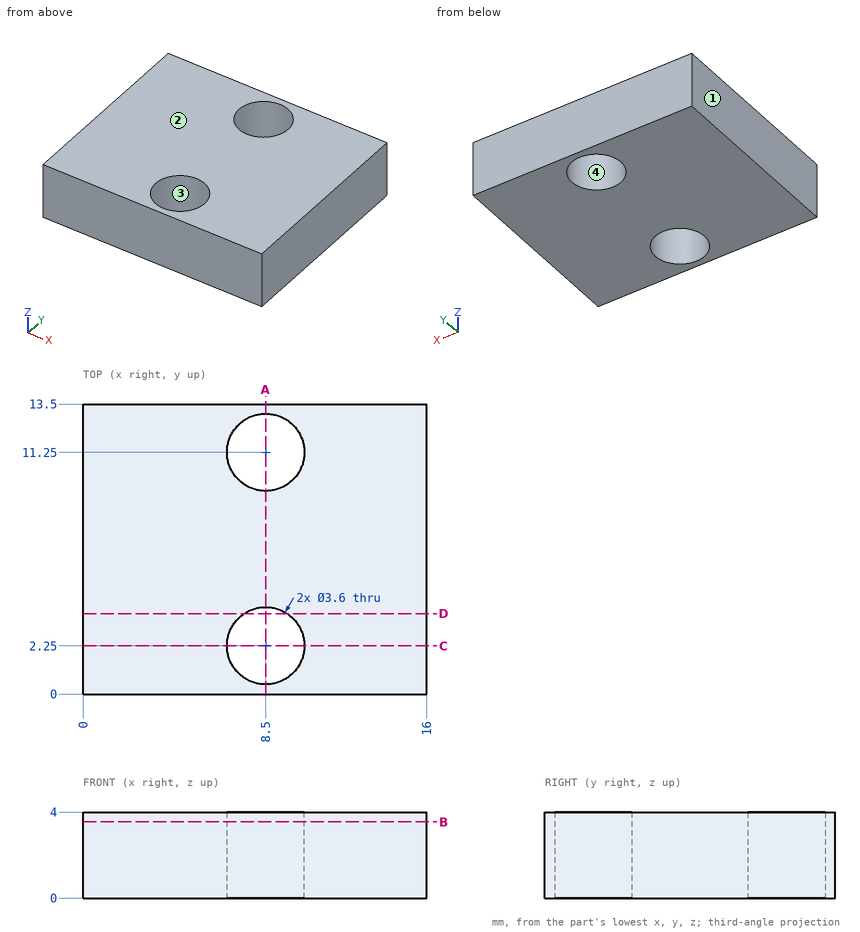
Geometry: see drawing. Coordinates: mm, zero at the bounding-box minimum. Round coordinates to 2 decimals unless told otherwise and drop trailing zeros. Loops run counter-clockwise (first coordinate to the right, second up) from the corner with the lowest first, then second, coordinate; pieces in that order, holes last. Notation, with made-up numbers: (-22, 54) -> (10, 54) arc R11 cw to (10, 63) -> close; hole circle Ø7 at (-34, 15). An arc over 180 degrees is marked (long way). Use one line per item in the form item = value. Start each with the question number.
Item 1: Material intervals for L1, parallel to Y at x = 9.5, z = 0.85; L2, parallel to X at y = 2.25, z = 1.85; L3, parallel to Y at x = 7.75, z = 0.6, sorted ascending. Write a range as from..to.
Item 2: Section query B-B on z = 3.55. Return the cut outline in (x, y).
Item 3: Section query C-C on y = 2.25. Return the cut outline in (x, z).
Item 4: Section query D-D on y = 3.75. Return the cut outline in (x, z).
Item 5: Mould query, pull axis X, two halves, no side actions, for the marked faces 1, 2, 3 and 4. Classes: pulls with the +X half, pulls with the -X half, needs draft (parallel to the pull), parting line crosses it, or undercut.
Item 6: Section query A-A on x = 8.5. Return the cut outline in (y, z).
Ans:
q1.L1 = 0..0.75, 3.75..9.75, 12.75..13.5
q1.L2 = 0..6.7, 10.3..16
q1.L3 = 0..0.61, 3.89..9.61, 12.89..13.5
q2.outline = (0, 0) -> (16, 0) -> (16, 13.5) -> (0, 13.5) -> close; hole circle Ø3.6 at (8.5, 2.25); hole circle Ø3.6 at (8.5, 11.25)
q3.outline = (0, 0) -> (6.7, 0) -> (6.7, 4) -> (0, 4) -> close; (10.3, 0) -> (16, 0) -> (16, 4) -> (10.3, 4) -> close
q4.outline = (0, 0) -> (7.51, 0) -> (7.51, 4) -> (0, 4) -> close; (9.49, 0) -> (16, 0) -> (16, 4) -> (9.49, 4) -> close
q5.face_1 = pulls with the -X half
q5.face_2 = needs draft
q5.face_3 = undercut
q5.face_4 = undercut
q6.outline = (0, 0) -> (0.45, 0) -> (0.45, 4) -> (0, 4) -> close; (4.05, 0) -> (9.45, 0) -> (9.45, 4) -> (4.05, 4) -> close; (13.05, 0) -> (13.5, 0) -> (13.5, 4) -> (13.05, 4) -> close
